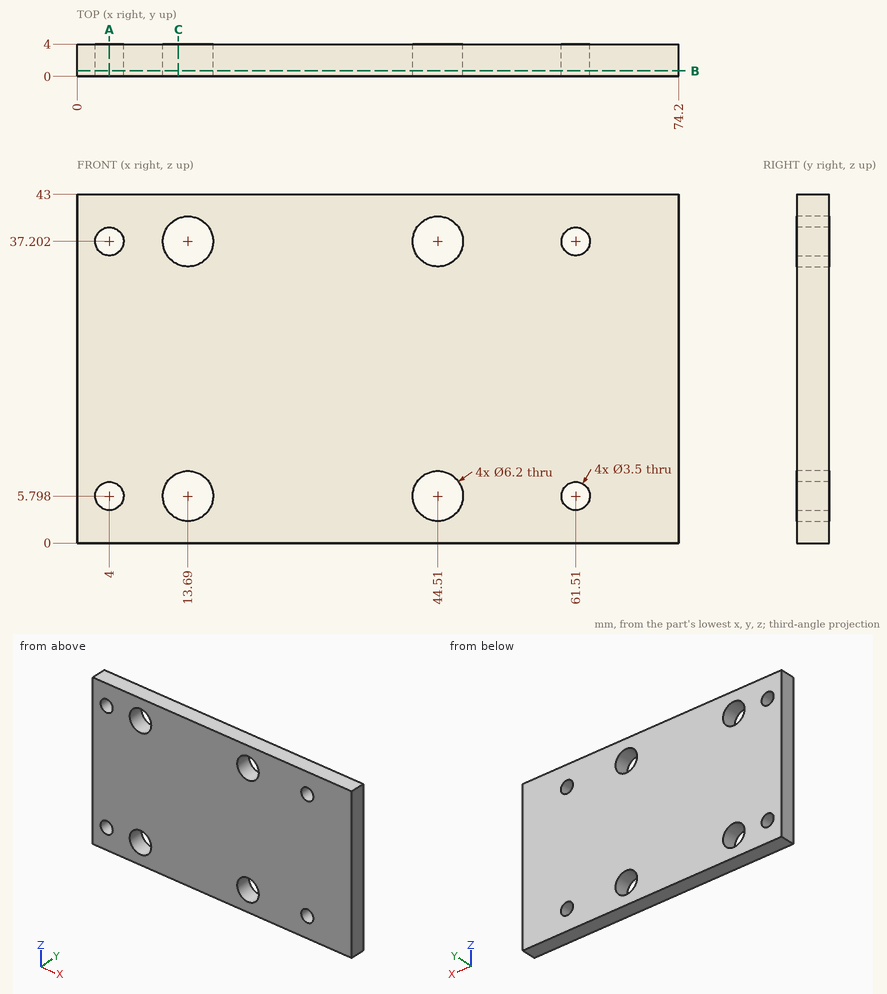
Verification items for this drawing (mm, ordinates from the low corner). Give positions to 0.01 mm unless a question says otherwise; leave off trailing zeros. Loops run counter-clockwise (first coordinate to the right, second up) from the corner with the lowest first, then second, coordinate; pieces in that order, holes last. Notation, with made-up numbers: M -9,7 L 45,7 A32 cw 45,35 Z; hole C 27.5,-30.5 d3. An arc over 180 degrees is marked long. Answer as a JSON object with one key per item and string values. Group by question number.
Item 1: Sectioned sample at A-A on x = 4. Record the boundary of the cut face in (y, z), plus the area to 3 significant figures.
Item 2: Material ranges on L1, parallel to X at y = 1.4, z = 3 (1 decimal); L2, parallel to Z at x = 16.5, y = 3 (1 decimal); L3, parallel to X at y = 2.55, z = 38.5 (1 decimal), recorded low to high.
Item 3: Sectioned sample at B-B on y = 0.7. Give the number of separate pieces and of enclosed holes in the cut face, plus the area to 3 significant figures.
Item 4: Sectioned sample at C-C on x = 12.5. Record the boundary of the cut face in (y, z).
Item 5: Gauge pin test, flat end, axial feed: pin 1 (5 mm diameter, centred on x = 13.69, z = 37.2, fed in from +Y). Record the tip position at first contact, or that the pin passes through.
Findings below:
{
 "1": {"outline": "M 0,0 L 4,0 L 4,4.05 L 0,4.05 Z; M 0,7.55 L 4,7.55 L 4,35.45 L 0,35.45 Z; M 0,38.95 L 4,38.95 L 4,43 L 0,43 Z", "area": "144 mm2"},
 "2": {"L1": "0 to 12.4, 15 to 43.2, 45.8 to 74.2", "L2": "0 to 4.5, 7.1 to 35.9, 38.5 to 43", "L3": "0 to 2.8, 5.2 to 10.9, 16.5 to 41.7, 47.3 to 60.3, 62.7 to 74.2"},
 "3": {"separate pieces": "1", "enclosed holes": "8", "area": "3,030 mm2"},
 "4": {"outline": "M 0,0 L 4,0 L 4,2.94 L 0,2.94 Z; M 0,8.66 L 4,8.66 L 4,34.34 L 0,34.34 Z; M 0,40.06 L 4,40.06 L 4,43 L 0,43 Z"},
 "5": {"pin 1": "through"}
}
